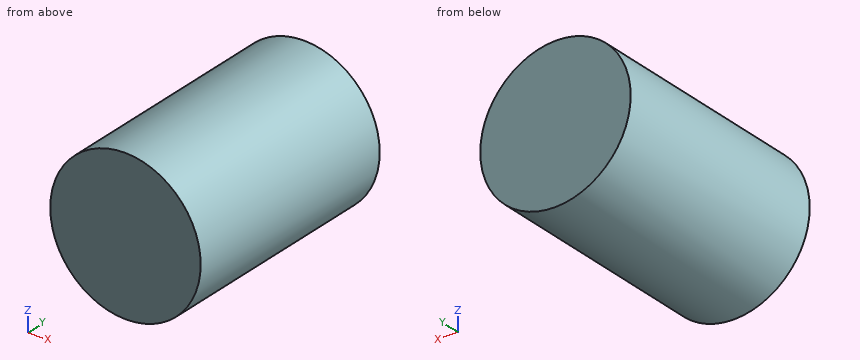
from build123d import *
from build123d.topology import SkipClean

# Parameters (mm, degrees)
SKETCH1_R               = 4.65
BOSS_EXTRUDE1_DEPTH     = 12
SKETCH2_R               = 17.5
BOSS_EXTRUDE2_DEPTH     = 2
SKETCH3_W               = 5
SKETCH3_H               = 13
BOSS_EXTRUDE3_DEPTH     = 12
FILLET1_R               = 4
FILLET2_R               = 4
CUT_EXTRUDE1_DEPTH      = 29.434134416
SKETCH5_R               = 2.05
CUT_EXTRUDE2_DEPTH      = 70
FILLET3_R               = 4
SKETCH6_R               = 24.65
SKETCH6_R_2             = 4.65
CUT_EXTRUDE_THIN1_DEPTH = 25.540782384
SKETCH7_R               = 24.575
SKETCH7_R_2             = 4.575
CUT_EXTRUDE_THIN2_DEPTH = 30


with BuildPart() as part:
    # Sketch1 → Boss-Extrude1 (new body)
    with BuildSketch(Plane(origin=(0, 0, 0), x_dir=(1, 0, 0), z_dir=(0, 1, 0))):
        with Locations(Location((0, 0, 0), (0, 0, 270))):
            Circle(SKETCH1_R)
    extrude(amount=BOSS_EXTRUDE1_DEPTH)

    # Sketch2 → Boss-Extrude2 (add)
    with BuildSketch(Plane(origin=(0, 12, 0), x_dir=(1, 0, 0), z_dir=(0, 1, 0))):
        with Locations(Location((0, 0, 0), (0, 0, 270))):
            Circle(SKETCH2_R)
    extrude(amount=BOSS_EXTRUDE2_DEPTH)

    # Sketch3 → Boss-Extrude3 (add)
    with BuildSketch(Plane(origin=(0, 14, 0), x_dir=(1, 0, 0), z_dir=(0, 1, 0))):
        with Locations((7.5, 0)):
            Rectangle(SKETCH3_W, SKETCH3_H)
    boss_extrude3 = extrude(amount=BOSS_EXTRUDE3_DEPTH)

    # Mirror1: Boss-Extrude3 across plane
    add(boss_extrude3.mirror(Plane(origin=(0, 0, 0), x_dir=(0, 0, 1), z_dir=(1, 0, 0))))

    # Fillet1
    fillet1_edges = [part.edges().sort_by_distance(p)[0] for p in [
        (7.5, 26, -6.5),
        (7.5, 26, 6.5),
        (-7.5, 26, 6.5),
        (-7.5, 26, -6.5),
    ]]
    fillet(fillet1_edges, radius=FILLET1_R)

    # Fillet2
    fillet2_edges = [part.edges().sort_by_distance(p)[0] for p in [
        (7.5, 14, 6.5),
        (7.5, 14, -6.5),
        (-7.5, 14, -6.5),
        (-7.5, 14, 6.5),
    ]]
    fillet(fillet2_edges, radius=FILLET2_R)

    # Sketch4 → Cut-Extrude1 (cut, through all)
    with BuildSketch(Plane(origin=(0, 14, 0), x_dir=(1, 0, 0), z_dir=(0, 1, 0))):
        with BuildLine():
            Line((10, 14.361406616), (10, 0))
            Line((10, 0), (10, -14.361406616))
            ThreePointArc((10, -14.361406616), (15.512092057, -8.100925873), (17.5, 0))
            ThreePointArc((17.5, 0), (15.512092057, 8.100925873), (10, 14.361406616))
        make_face()
    cut_extrude1 = extrude(amount=-CUT_EXTRUDE1_DEPTH, mode=Mode.SUBTRACT)

    # Mirror2: Cut-Extrude1 across plane
    add(cut_extrude1.mirror(Plane(origin=(0, 0, 0), x_dir=(0, 0, 1), z_dir=(1, 0, 0))), mode=Mode.SUBTRACT)

    # Sketch5 → Cut-Extrude2 (cut)
    with BuildSketch(Plane(origin=(10, 0, 0), x_dir=(0, 0, -1), z_dir=(1, 0, 0))):
        with Locations((0, 20)):
            Circle(SKETCH5_R)
    extrude(amount=-CUT_EXTRUDE2_DEPTH, mode=Mode.SUBTRACT)

    # Fillet3
    fillet3_edges = [part.edges().sort_by_distance(p)[0] for p in [
        (10, 13, -14.361406616),
        (10, 13, 14.361406616),
        (-10, 13, 14.361406616),
        (-10, 13, -14.361406616),
    ]]
    fillet(fillet3_edges, radius=FILLET3_R)

    # Sketch6 → Cut-Extrude-Thin1 (cut, through all)
    with SkipClean():  # the faces are left unmerged after this step: merging them gives an invalid solid
        with BuildSketch(Plane.XZ.offset(-12)):
            Circle(SKETCH6_R)
            Circle(SKETCH6_R_2, mode=Mode.SUBTRACT)
        extrude(amount=-CUT_EXTRUDE_THIN1_DEPTH, mode=Mode.SUBTRACT)

    # Sketch7 → Cut-Extrude-Thin2 (cut)
    with BuildSketch(Plane(origin=(0, 14, 0), x_dir=(1, 0, 0), z_dir=(0, 1, 0))):
        Circle(SKETCH7_R)
        Circle(SKETCH7_R_2, mode=Mode.SUBTRACT)
    extrude(amount=-CUT_EXTRUDE_THIN2_DEPTH, mode=Mode.SUBTRACT)


solid = part.part
Can you work these out from the model? Positions are in its coordinate system, mm. Give positions to 0.01 mm unless a question says otherwise; leave off trailing zeros. Loops run counter-clockwise (first coordinate to the right, second up) from the corner with the lowest first, then second, coordinate; pieces in that order, holes last. Notation, with made-up numbers: (-1, -17) -> (4, -17) arc R16 ccw to (4, -12) -> close; hole circle Ø6 at (68.25, 3). An arc over 180 degrees is marked (long way). Write item = value, one per line.
1) I need wall thicknesses on L1, parallel to Z at x = -3, y = 5.5; L2, parallel to X at y = 4.5, z = -1. Which ranges of each line are inside material? Lowest first, please. Write a range as from..to.
Check result:
L1 = -3.45..3.45
L2 = -4.46..4.46
2) Will this pin go through, and if not, where does the flat tip stop? pin 1 (3 mm diameter, centred on x = -0.5, y = 3.5, fed in from +Z) (3 decimals).
Check result:
pin_1 = 4.575
3) Suppose I cut it at B-B on x = -1.75. Write out the boundary of the cut face in (y, z).
Check result:
outline = (0, -4.23) -> (14, -4.23) -> (14, 4.23) -> (0, 4.23) -> close
4) Suppose I cut it at A-A on y = 7.25. Write out the boundary of the cut face in (x, z) (3 decimals), then the cut area to 3 significant figures.
Check result:
outline = circle Ø9.15 at (0, 0)
area = 65.8 mm2
5) Suppose I cut it at C-C on z = -3. Write out the boundary of the cut face in (x, y).
Check result:
outline = (-3.45, 0) -> (3.45, 0) -> (3.45, 14) -> (-3.45, 14) -> close
